Build history of the part. All positions in model axes, mm. A direction names the side the tool comes from. Round coordinates to 2 decimals unless told otherwise and drop trailing zeros. Return JSON: item names as keys, results as strings.
from build123d import *

# Parameters (mm, degrees)
F1_W          = 40
F1_H          = 40
F2_DEPTH      = 250
F3_R          = 4
F3_R_2        = 3.4
F4_DEPTH      = 250.001
F4_DEPTH_BACK = 250.001
F6_DEPTH      = 250.001
F6_DEPTH_BACK = 250.001
F7_R          = 1


with BuildPart() as f2:
    # F1 (on Front) → F2 (new body, symmetric)
    with BuildSketch(Plane.XZ):
        Rectangle(F1_W, F1_H)
    extrude(amount=F2_DEPTH, both=True)

    # F3 (on Front) → F4 (cut, two sides)
    with BuildSketch(Plane.XZ) as f4_sk:
        with Locations((-13.5, 13.5)):
            Circle(F3_R)
        with Locations((-13.5, -13.5)):
            Circle(F3_R)
        with Locations((13.5, -13.5)):
            Circle(F3_R)
        with Locations((13.5, 13.5)):
            Circle(F3_R)
        Circle(F3_R_2)
    extrude(amount=-F4_DEPTH, mode=Mode.SUBTRACT)
    extrude(f4_sk.sketch, amount=F4_DEPTH_BACK, mode=Mode.SUBTRACT)

    # F5 (on Front) → F6 (cut, two sides)
    with BuildSketch(Plane.XZ) as f6_sk:
        with BuildLine():
            Line((4.2, 20), (-4.2, 20))
            Line((-4.2, 20), (-4.2, 16))
            Line((-4.2, 16), (-7.25, 16))
            Line((-7.25, 16), (-7.25, 8.8609854211))
            ThreePointArc((-7.25, 8.8609854211), (0, 5.5), (7.25, 8.8609854211))
            Line((7.25, 8.8609854211), (7.25, 16))
            Line((7.25, 16), (4.2, 16))
            Line((4.2, 16), (4.2, 20))
        make_face()
        with BuildLine():
            Line((-16, 7.25), (-16, 4.2))
            Line((-16, 4.2), (-20, 4.2))
            Line((-20, 4.2), (-20, -4.2))
            Line((-20, -4.2), (-16, -4.2))
            Line((-16, -4.2), (-16, -7.25))
            Line((-16, -7.25), (-8.8609854211, -7.25))
            ThreePointArc((-8.8609854211, -7.25), (-5.5, 0), (-8.8609854211, 7.25))
            Line((-8.8609854211, 7.25), (-16, 7.25))
        make_face()
        with BuildLine():
            Line((-7.25, -16), (-4.2, -16))
            Line((-4.2, -16), (-4.2, -20))
            Line((-4.2, -20), (4.2, -20))
            Line((4.2, -20), (4.2, -16))
            Line((4.2, -16), (7.25, -16))
            Line((7.25, -16), (7.25, -8.8609854211))
            ThreePointArc((7.25, -8.8609854211), (0, -5.5), (-7.25, -8.8609854211))
            Line((-7.25, -8.8609854211), (-7.25, -16))
        make_face()
        with BuildLine():
            Line((16, -7.25), (16, -4.2))
            Line((16, -4.2), (20, -4.2))
            Line((20, -4.2), (20, 4.2))
            Line((20, 4.2), (16, 4.2))
            Line((16, 4.2), (16, 7.25))
            Line((16, 7.25), (8.8609854211, 7.25))
            ThreePointArc((8.8609854211, 7.25), (5.5, 0), (8.8609854211, -7.25))
            Line((8.8609854211, -7.25), (16, -7.25))
        make_face()
    extrude(amount=-F6_DEPTH, mode=Mode.SUBTRACT)
    extrude(f6_sk.sketch, amount=F6_DEPTH_BACK, mode=Mode.SUBTRACT)

    # F7
    f7_edges = [f2.edges().sort_by_distance(p)[0] for p in [
        (-20, 0, 20),
        (20, 0, 20),
        (20, 0, -20),
        (-20, 0, -20),
    ]]
    fillet(f7_edges, radius=F7_R)


solid = f2.part
Q1. 3-axis set-ups, long thin cutter, end or side, ignore diameter. For faces 4 (the flat face through (20, -4, -12)), 5 (the cylindrical face through (-5.5, 3.5, -0.1)): which of +Z, -Z, +X, -X, +Y, -Y reach the whole face in a straight line?
Verdict:
{"face 4": "+Z, -Z, +X, +Y, -Y", "face 5": "+Y, -Y"}
Q2. Saw through at A-A on y = 53. Count the separate pieces of the cut face and the enclosed holes in it, then the cut area to 3 significant figures.
Verdict:
{"separate pieces": "1", "enclosed holes": "5", "area": "678 mm²"}
Q3. Wall check: L1, parallel to X at y = 28, z = -13; L2, parallel to Z at x = 13.5, y = -56.5; L3, parallel to Z at x = 11, y = -205. Give the ranges that are in metal, low to high.
Verdict:
{"L1": "x = -20 to -17.47, -9.53 to -7.25, 7.25 to 9.53, 17.47 to 20", "L2": "z = -20 to -17.5, -9.5 to -7.25, 7.25 to 9.5, 17.5 to 20", "L3": "z = -20 to -16.62, -10.38 to -7.25, 7.25 to 10.38, 16.62 to 20"}
Q4. Two-plate mould, pull along X, no slides. Class faces 1 (the flat face through (11, -4, 20)), 2 (the flat face through (-20, -4, -12)), 3 (the cylindrical face through (-0.1, 3.5, 5.5)): +X half, -X half, draft (parallel to the pull), parting line (faces both ways), or undercut.
Verdict:
{"face 1": "draft", "face 2": "-X half", "face 3": "undercut"}
